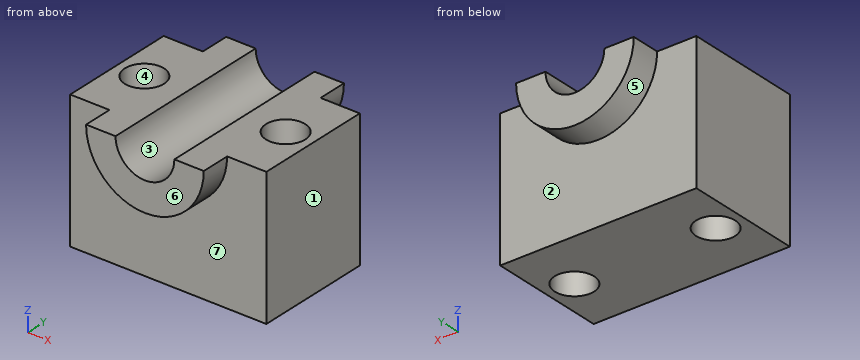
from build123d import *

# Parameters (mm, degrees)
F0_W     = 127
F0_H     = 76.2
F1_DEPTH = 88.9
F2_R     = 38.1
F3_DEPTH = 57.15
F5_DEPTH = 127
F6_R     = 19.05
F7_DEPTH = 127
F8_R     = 12.7
F9_DEPTH = 88.901


with BuildPart() as f1:
    # F0 (on Top) → F1 (new body)
    with BuildSketch(Plane.XY):
        Rectangle(F0_W, F0_H)
    extrude(amount=F1_DEPTH)

    # F2 (on Front) → F3 (join, symmetric)
    with BuildSketch(Plane.XZ):
        with Locations((0, 88.9)):
            Circle(F2_R)
    extrude(amount=F3_DEPTH, both=True)

    # F4 (on Front) → F5 (cut, symmetric)
    with BuildSketch(Plane.XZ):
        with BuildLine():
            Line((76.654768, 131.578267), (-50.806063, 131.578267))
            Line((-50.806063, 131.578267), (-50.806063, 88.9))
            Line((-50.806063, 88.9), (-19.05, 88.9))
            ThreePointArc((-19.05, 88.9), (0, 107.95), (19.05, 88.9))
            Line((19.05, 88.9), (76.654768, 88.9))
            Line((76.654768, 88.9), (76.654768, 131.578267))
        make_face()
    extrude(amount=F5_DEPTH, both=True, mode=Mode.SUBTRACT)

    # F6 (on Front) → F7 (cut, symmetric)
    with BuildSketch(Plane.XZ):
        with Locations((0, 88.9)):
            Circle(F6_R)
    extrude(amount=F7_DEPTH, both=True, mode=Mode.SUBTRACT)

    # F8 (on face) → F9 (cut, through all)
    with BuildSketch(Plane.XY.offset(88.9)):
        with Locations((-45.72, 0)):
            Circle(F8_R)
        with Locations((45.72, 0)):
            Circle(F8_R)
    extrude(amount=-F9_DEPTH, mode=Mode.SUBTRACT)


solid = f1.part
Design review of the part built by this model. Coordinates are the model's own, in mm. Face numbers are marked on the shaded views. A direction names the side the tool comes from. Round coordinates to 2 decimals unless told otherwise and drop trailing zeros. Order: outer loops, then holes, each group sorted by start corner. A loop starts at its lowest first (then second) coordinate and runs counter-clockwise, first axis right, second up.
1) Draft analysis for pull direction X (two halves, no side actions). For the marked faces 1, 2, 3 and 4, state which applies: released by +X, released by -X, zero draft, split by the parting line, or undercut.
The answers:
face 1: released by +X
face 2: zero draft
face 3: undercut
face 4: undercut
2) Consider section C-C (z = 40). State the section outline as (x, y) points, plus the area to 3 significant figures.
The answers:
outline: (-63.5, -38.1) - (63.5, -38.1) - (63.5, 38.1) - (-63.5, 38.1) - close; hole circle Ø25.4 at (-45.72, 0); hole circle Ø25.4 at (45.72, 0)
area: 8,660 mm2
3) Clearance check with flat-ended pins moving along their axes: pin 1 Ø6 at (x, y) = (23.5, 21) entering from -Z; pin 2 Ø10 at (x, z) = (10, 40) entering from +Y; pin 3 Ø4 at (x, z) = (34, 18) entering from -Y. State where each tip first meets the part, or that it passes through.
The answers:
pin 1: stops at z = 0
pin 2: stops at y = 38.1
pin 3: stops at y = -38.1
4) Consider section A-A (x = 45.72). State the section outline as (y, z) points, plus the area to 3 significant figures.
The answers:
outline: (-38.1, 0) - (-12.7, 0) - (-12.7, 88.9) - (-38.1, 88.9) - close; (12.7, 0) - (38.1, 0) - (38.1, 88.9) - (12.7, 88.9) - close
area: 4,520 mm2
5) For L1, parallel to Y at x = -45, z = 18; L2, parallel to X at y = 5, z = 72; L3, parallel to X at y = -6.5, z = 25, list the stretches that pass through material, from the lowest coordinate up.
The answers:
L1: y = -38.1 to -12.68, 12.68 to 38.1
L2: x = -63.5 to -57.39, -34.05 to -8.79, 8.79 to 34.05, 57.39 to 63.5
L3: x = -63.5 to -56.63, -34.81 to 34.81, 56.63 to 63.5
6) Machinability: for the marked faces 5, 6 and 7, which of the approach directions +Z, -Z, +X, -X, +Y, -Y give a long, thin tool a straight path to every point of the face, cutting with its end or side? Answer none if there is none.
The answers:
face 5: -Z, +Y
face 6: +Z, -Z, +X, -X, -Y
face 7: -Z, -Y
7) Consider section B-B (y = -6). State the section outline as (x, z) points.
The answers:
outline: (-63.5, 0) - (-56.91, 0) - (-56.91, 88.9) - (-63.5, 88.9) - close; (-34.53, 0) - (34.53, 0) - (34.53, 88.9) - (19.05, 88.9) arc R19.05 cw to (-19.05, 88.9) - (-34.53, 88.9) - close; (56.91, 0) - (63.5, 0) - (63.5, 88.9) - (56.91, 88.9) - close
8) Consider section D-D (y = -28.5). State the section outline as (x, z) points.
The answers:
outline: (-63.5, 0) - (63.5, 0) - (63.5, 88.9) - (19.05, 88.9) arc R19.05 cw to (-19.05, 88.9) - (-63.5, 88.9) - close
